from build123d import *

# Parameters (mm, degrees)
SKETCH2_W               = 55
SKETCH2_H               = 38
BOSS_EXTRUDE1_DEPTH     = 2
SKETCH3_R               = 3.2
BOSS_EXTRUDE2_DEPTH     = 10
SKETCH4_R               = 3.6
BOSS_EXTRUDE3_DEPTH     = 1
CHAMFER1_SIZE           = 3
SKETCH5_W               = 2
SKETCH5_H               = 10.684354826
CUT_EXTRUDE1_DEPTH      = 6
CHAMFER2_SIZE           = 10
CUT_EXTRUDE2_DEPTH      = 35.889110049
CUT_EXTRUDE2_DEPTH_BACK = 35.889110049
SKETCH8_W               = 9.45
SKETCH8_H               = 2
SKETCH9_R               = 3
BOSS_EXTRUDE4_DEPTH     = 5.75
FILLET1_R               = 4
FILLET2_R               = 16


with BuildPart() as part:
    # Sketch2 → Boss-Extrude1 (new body)
    with BuildSketch(Plane(origin=(0, 0, 0), x_dir=(1, 0, 0), z_dir=(0, 1, 0))):
        Rectangle(SKETCH2_W, SKETCH2_H)
    extrude(amount=BOSS_EXTRUDE1_DEPTH)

    # Sketch3 → Boss-Extrude2 (add)
    with BuildSketch(Plane(origin=(0, 0, 0), x_dir=(1, 0, 0), z_dir=(0, 1, 0))):
        with Locations(Location((-16.675, 3.65, 0), (0, 0, 270))):
            Circle(SKETCH3_R)
        with Locations(Location((16.675, 3.65, 0), (0, 0, 90))):
            Circle(SKETCH3_R)
    extrude(amount=BOSS_EXTRUDE2_DEPTH)

    # Sketch4 → Boss-Extrude3 (add)
    with BuildSketch(Plane(origin=(0, 10, 0), x_dir=(1, 0, 0), z_dir=(0, 1, 0))):
        with Locations(Location((-16.675, 3.65, 0), (0, 0, 270))):
            Circle(SKETCH4_R)
        with Locations(Location((16.675, 3.65, 0), (0, 0, 90))):
            Circle(SKETCH4_R)
    extrude(amount=-BOSS_EXTRUDE3_DEPTH)

    # Chamfer1
    # the kernel refuses this chamfer: 3 mm, written as the material it adds along each edge
    with BuildSketch(Plane(origin=(16.675, 9, -3.65), x_dir=(0, 0, -1), z_dir=(-1, 0, 0))) as chamfer1_piece_1_section:
        Polygon((3.2, CHAMFER1_SIZE), (3.2 + CHAMFER1_SIZE, 0), (3.2, 0), align=None)
    chamfer1_piece_1 = revolve(axis=Axis((16.675, 9, -3.65), (0, -1, 0)), mode=Mode.PRIVATE)
    chamfer1_piece_1 = chamfer1_piece_1 & Plane(origin=(16.675, 6.179265151, -3.65), x_dir=(0, 0, -1), z_dir=(0, 1, 0)) * Cylinder(3.6, 25, mode=Mode.PRIVATE)
    add(chamfer1_piece_1)
    with BuildSketch(Plane(origin=(-16.675, 9, -3.65), x_dir=(0, 0, 1), z_dir=(1, 0, 0))) as chamfer1_piece_2_section:
        Polygon((3.2, CHAMFER1_SIZE), (3.2 + CHAMFER1_SIZE, 0), (3.2, 0), align=None)
    chamfer1_piece_2 = revolve(axis=Axis((-16.675, 9, -3.65), (0, -1, 0)), mode=Mode.PRIVATE)
    chamfer1_piece_2 = chamfer1_piece_2 & Plane(origin=(-16.675, 6.179265151, -3.65), x_dir=(0, 0, 1), z_dir=(0, 1, 0)) * Cylinder(3.6, 25, mode=Mode.PRIVATE)
    add(chamfer1_piece_2)

    # Sketch5 → Cut-Extrude1 (cut)
    with BuildSketch(Plane(origin=(0, 10, 0), x_dir=(1, 0, 0), z_dir=(0, 1, 0))):
        with Locations((16.675, 3.65)):
            Rectangle(SKETCH5_W, SKETCH5_H)
        with Locations((-16.675, 3.65)):
            Rectangle(SKETCH5_W, SKETCH5_H)
    extrude(amount=-CUT_EXTRUDE1_DEPTH, mode=Mode.SUBTRACT)

    # Chamfer2
    chamfer2_edges = [part.edges().sort_by_distance(p)[0] for p in [
        (-27.5, 1, -19),
        (27.5, 1, -19),
    ]]
    chamfer(chamfer2_edges, length=CHAMFER2_SIZE)

    # Sketch8 → Cut-Extrude2 (cut, two sides: drawn at the far end of the back side and taken through both)
    with BuildSketch(Plane.ZY.offset(-CUT_EXTRUDE2_DEPTH_BACK)):
        with Locations((14.275, 1)):
            Rectangle(SKETCH8_W, SKETCH8_H)
    extrude(amount=CUT_EXTRUDE2_DEPTH + CUT_EXTRUDE2_DEPTH_BACK, mode=Mode.SUBTRACT)

    # Sketch9 → Boss-Extrude4 (add, symmetric)
    with BuildSketch(Plane.ZY):
        with BuildLine():
            Line((9.55, 2), (11.05, 4.828427125))
            ThreePointArc((11.05, 4.828427125), (19.792640687, 6.328427125), (12.05, 2))
            Line((12.05, 2), (9.55, 0))
            Line((9.55, 0), (9.55, 2))
        make_face()
        with Locations((15.55, 4.828427125)):
            Circle(SKETCH9_R, mode=Mode.SUBTRACT)
    extrude(amount=BOSS_EXTRUDE4_DEPTH, both=True)

    # Fillet1
    fillet1_edges = [part.edges().sort_by_distance(p)[0] for p in [
        (0, 2, 9.55),
        (0, 2, 12.05),
    ]]
    fillet(fillet1_edges, radius=FILLET1_R)

    # Fillet2
    fillet2_edges = [part.edges().sort_by_distance(p)[0] for p in [
        (27.5, 1, 9.55),
        (-27.5, 1, 9.55),
    ]]
    fillet(fillet2_edges, radius=FILLET2_R)


solid = part.part
Verification items for the finished model (mm, model axes). A direction names the side the tool comes from. Round coordinates to 2 decimals unless told otherwise and drop trailing zeros. Loops run counter-clockwise (first coordinate to the right, second up) from the corner with the lowest first, then second, coordinate; pieces in that order, holes last. Notation, with made-up numbers: M 4.25,26.25 L 13.25,26.25 A16 cw 13.25,54.25 Z; hole C -1.75,-34 d10. An arc over 180 degrees is marked long. Write each question's results on one line, items separated by ' | '.
1) Section check B-B on y = 7.25. Record the boundary of the cut face in (x, z) (3 decimals).
Checks:
outline: M -17.675,-7.108 L -17.675,-0.192 A3.6 ccw Z; M -15.675,-7.108 A3.6 ccw -15.675,-0.192 Z; M -5.75,11.757 L 5.75,11.757 L 5.75,13.779 L -5.75,13.779 Z; M -5.75,17.321 L 5.75,17.321 L 5.75,19.343 L -5.75,19.343 Z; M 15.675,-7.108 L 15.675,-0.192 A3.6 ccw Z; M 17.675,-7.108 A3.6 ccw 17.675,-0.192 Z
2) Section check D-D on x = 9. Record the boundary of the cut face in (y, z).
Checks:
outline: M 0,-19 L 2,-19 L 2,9.55 L 0,9.55 Z
3) Section check A-A on z = 15.55. Record the boundary of the cut face in (x, y), then the cut area to 3 significant figures.
Checks:
outline: M -5.75,0.33 L 5.75,0.33 L 5.75,1.83 L -5.75,1.83 Z; M -5.75,7.83 L 5.75,7.83 L 5.75,9.33 L -5.75,9.33 Z | area: 34.5 mm2
4) Section check C-C on x = 0. Record the boundary of the cut face in (y, z).
Checks:
outline: M 0,-19 L 2,-19 L 2,7.14 A4 cw 4.13,10.68 L 4.83,11.05 A4.5 ccw long 0.69,13.78 A4 cw 0.13,9.72 L 0,9.55 Z; hole C 4.83,15.55 d6
5) Scan lines: L1, parallel to X at y = 8, z = -2 (3 decimals); L2, parallel to X at y = 5, z = -5 (3 decimals); L3, parallel to Y at x = -3.5, z = 15.55. Record each from-to range of solid material in increasing order. Write a range as from..to.
Checks:
L1: x = -19.875..-17.675, -15.675..-13.475, 13.475..15.675, 17.675..19.875 | L2: x = -19.576..-17.675, -15.675..-13.774, 13.774..15.675, 17.675..19.576 | L3: y = 0.33..1.83, 7.83..9.33
6) Access from +Z, -Z, +X, -X, +Y, -Y to the whole of each face (thin tool, end or side, straight path). Record for faces 5 (the cylindrical face through (-22.689, 0.986, 4.987)), 6 (the flat face through (9, 1, 9.55)), 7 (the flat face through (-17, 4, -4)), 8 (the conical face through (13.362, 6.114, -3.59)), 9 (the cylindrical face through (-13.076, 8.225, -3.585)).
Checks:
face 5: +Z, -X, +Y, -Y | face 6: +Z, +X, +Y, -Y | face 7: +Z, -Z, +Y | face 8: none | face 9: +Y
7) Gauge pin test, flat ends, axial feed: P1, Ø1, axis at x = -17, z = -4.5, coming from the +Y side; P2, Ø8.5, axis at x = 3.5, z = -5.5, coming from the +Y side; P3, Ø4, axis at x = 3.5, y = 4.5, coming from the -Z side. Record the tip position at first contact, or that the pin passes through.
Checks:
P1: stops at y = 4 | P2: stops at y = 2 | P3: stops at z = 9.08
8) Mould release check, pull along Z, two halves, no side actions. Record for faces 1 (the flat face through (19, 10, -4)), 2 (the cylindrical face through (0.08, 2.167, 16.934)), 3 (the flat face through (-9, 1, 9.55)), 4 (the flat face through (0, 1, -19)): released by +Z, released by -Z, zero draft, split by the parting line, or undercut.
Checks:
face 1: zero draft | face 2: undercut | face 3: released by +Z | face 4: released by -Z
